The figure shows three views and two pictorial views of one solid part (mm, origin at its lowest corner). Answer the questions. A direction names the side the tool comes from. Round coordinates to 2 decimals unless told otherwise and drop trailing zeros. Write each loop counter-clockwise with the first axis right and the second up, starting at its lowest first coordinate (ties: lowest second). Pieces come first, ordered by that corner, then holes.
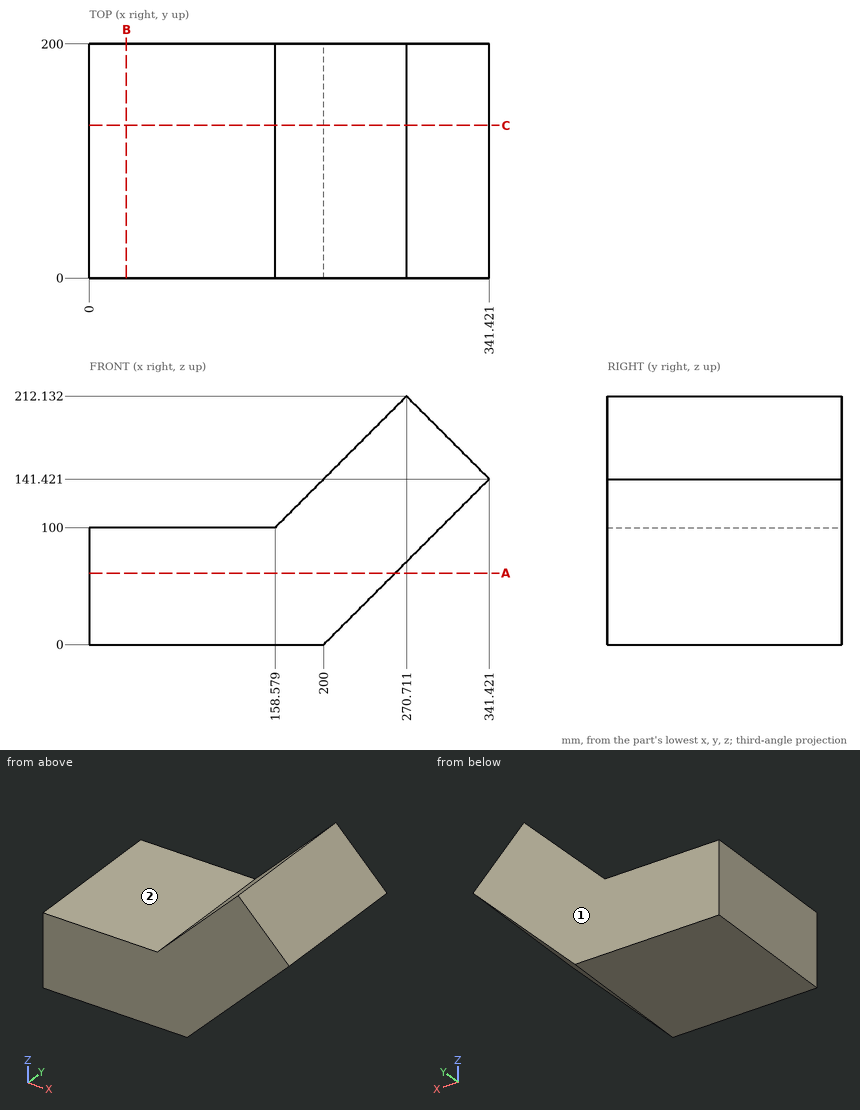
Q1. Flat-ended cylindrical pins translate along their axes: pin 1 Ø5 at (y, z) = (69.5, 114.5) entering from +X; pin 2 Ø8 at (y, z) = (110, 135.5) entering from +X. Find the tip coordinate at first contact, or state that the pin passes through.
Verdict:
pin 1: stops at x = 317
pin 2: stops at x = 339.5
Q2. Section A-A (z = 61) is taken. Determine the outline of the cut face in (x, y).
Verdict:
outline: (0, 0) - (261, 0) - (261, 200) - (0, 200) - close
Q3. Which of the six approach directions +Z, -Z, +X, -X, +Y, -Y give full straight-line access (tool end or side, diameter ignored) to the marked faces 1 and 2?
Verdict:
face 1: +Z, -Z, +X, -X, +Y
face 2: +Z, -X, +Y, -Y
Q4. Section B-B (x = 31.5) is taken. Determine the outline of the cut face in (y, z), then the cut area to 3 significant figures.
Verdict:
outline: (0, 0) - (200, 0) - (200, 100) - (0, 100) - close
area: 20,000 mm2
Q5. Section C-C (y = 130.5) is taken. Determine the outline of the cut face in (x, z), then the cut area to 3 significant figures.
Verdict:
outline: (0, 0) - (200, 0) - (341.42, 141.42) - (270.71, 212.13) - (158.58, 100) - (0, 100) - close
area: 35,900 mm2
Q6. Straight lines are drawn through the part: probe 1 along Z at (x, y) = (64.5, 100); probe 2 along X at (y, z) = (123.5, 125); probe 3 along X at (y, z) = (60, 18). For each, find the intervals that lie inside material, in ascending order.
Verdict:
probe 1: z = 0 to 100
probe 2: x = 183.58 to 325
probe 3: x = 0 to 218
